from build123d import *

# Parameters (mm, degrees)
ESQUISSE1_W        = 230
ESQUISSE1_H        = 210
ESQUISSE1_R        = 1.5
ESQUISSE1_W_2      = 5
ESQUISSE1_H_2      = 5
BOSS_EXTRU_1_DEPTH = 5
CONG_1_R           = 5


with BuildPart() as part:
    # Esquisse1 → Boss.-Extru.1 (new body)
    with BuildSketch(Plane.XY):
        Rectangle(ESQUISSE1_W, ESQUISSE1_H)
        with Locations((107.5, 80)):
            Circle(ESQUISSE1_R, mode=Mode.SUBTRACT)
        with Locations((107.5, -80)):
            Circle(ESQUISSE1_R, mode=Mode.SUBTRACT)
        with Locations(Location((-107.5, -80, 0), (0, 0, 180))):
            Circle(ESQUISSE1_R, mode=Mode.SUBTRACT)
        with Locations(Location((-107.5, 80, 0), (0, 0, 180))):
            Circle(ESQUISSE1_R, mode=Mode.SUBTRACT)
        with Locations((107.5, 72.5)):
            Rectangle(ESQUISSE1_W_2, ESQUISSE1_H_2, mode=Mode.SUBTRACT)
        with Locations((107.5, 87.5)):
            Rectangle(ESQUISSE1_W_2, ESQUISSE1_H_2, mode=Mode.SUBTRACT)
        with Locations((107.5, -87.5)):
            Rectangle(ESQUISSE1_W_2, ESQUISSE1_H_2, mode=Mode.SUBTRACT)
        with Locations((107.5, -72.5)):
            Rectangle(ESQUISSE1_W_2, ESQUISSE1_H_2, mode=Mode.SUBTRACT)
        with Locations((-107.5, -87.5)):
            Rectangle(ESQUISSE1_W_2, ESQUISSE1_H_2, mode=Mode.SUBTRACT)
        with Locations((-107.5, -72.5)):
            Rectangle(ESQUISSE1_W_2, ESQUISSE1_H_2, mode=Mode.SUBTRACT)
        with Locations((-107.5, 72.5)):
            Rectangle(ESQUISSE1_W_2, ESQUISSE1_H_2, mode=Mode.SUBTRACT)
        with Locations((-107.5, 87.5)):
            Rectangle(ESQUISSE1_W_2, ESQUISSE1_H_2, mode=Mode.SUBTRACT)
    extrude(amount=BOSS_EXTRU_1_DEPTH)

    # Congé1
    cong_1_edges = [part.edges().sort_by_distance(p)[0] for p in [
        (-115, 105, 2.5),
        (115, 105, 2.5),
        (115, -105, 2.5),
        (-115, -105, 2.5),
    ]]
    fillet(cong_1_edges, radius=CONG_1_R)


solid = part.part
The model under review builds one solid part; all positions refer to its coordinate system, in mm. A direction names the side the tool comes from. Round coordinates to 2 decimals unless told otherwise and drop trailing zeros. Write item = value, one per line. Start each with the question number.
Item 1: For faces 4 (the face through (-115, -1, 2)), 5 (the face through (-108, 90, 2)), list the 3-axis set-ups (+Z, -Z, +X, -X, +Y, -Y) from which the entire face can be reached by the end or side of a thin tool; tool diameter is ignored.
Item 2: Mouldability with a two-part tool opening along Y and no side actions: class faces 1 (the face through (-108, 85, 2)), 2 (the face through (-2, 1, 0)), 3 (the face through (113, 104, 3)) as released by +Y, released by -Y, zero draft, split by the parting line, or undercut.
Item 3: For line 1 along X through (y, z) = (-80, 2.2), list the stretches that pass through material, from the lowest coordinate up.
Conclusion:
q1.face_4 = +Z, -Z, -X, +Y, -Y
q1.face_5 = +Z, -Z
q2.face_1 = undercut
q2.face_2 = zero draft
q2.face_3 = released by +Y
q3.line_1 = -115 to -109, -106 to 106, 109 to 115
